Geometry: see drawing. Coordinates: mm, zero at the bounding-box minimum. Give positions to 0.01 mm unless a question says otherwise; leave off trailing zeros. Write each loop counter-clockwise with the first axis right and the second up, starting at its lowest first coordinate (ties: lowest second). Pieces come first, ordered by that corner, then holes. Notation, with made-up numbers: M -24,-38 L -17,-38 A7 ccw -17,-28 Z; hole C 21,67.5 d10. An arc over 180 degrees is marked long. Use a Markdown table: item, result. Add a question column.
1) Section A-A on y = 6. Return the cut outline in (x, z).
2) Section B-B on x = 47. Return the cut outline in (y, z).
3) Pin query (flat end, axial travel): pin 1 (4 mm diameter, centred on y = 4.5, z = 37.5, fed in from -X); pin 2 (2.5 mm diameter, centred on x = 4.5, y = 3.5, fed in from +Z); pin 3 (2.5 mm diameter, centred on x = 97.5, y = 2.5, fed in from -Z). Return the tip coordinate at first contact, or that it passes through.
4) Line query: line 1 (X direction, y = 6.75, z = 55.5); line 2 (Z direction, x = 93, y = 6); line 3 (Z direction, x = 59.5, y = 1.75). Output: solid intervals per line, ascending.
5) Section C-C on z = 156.5. Return the cut outline in (x, y), then the cut area to 3 significant figures.
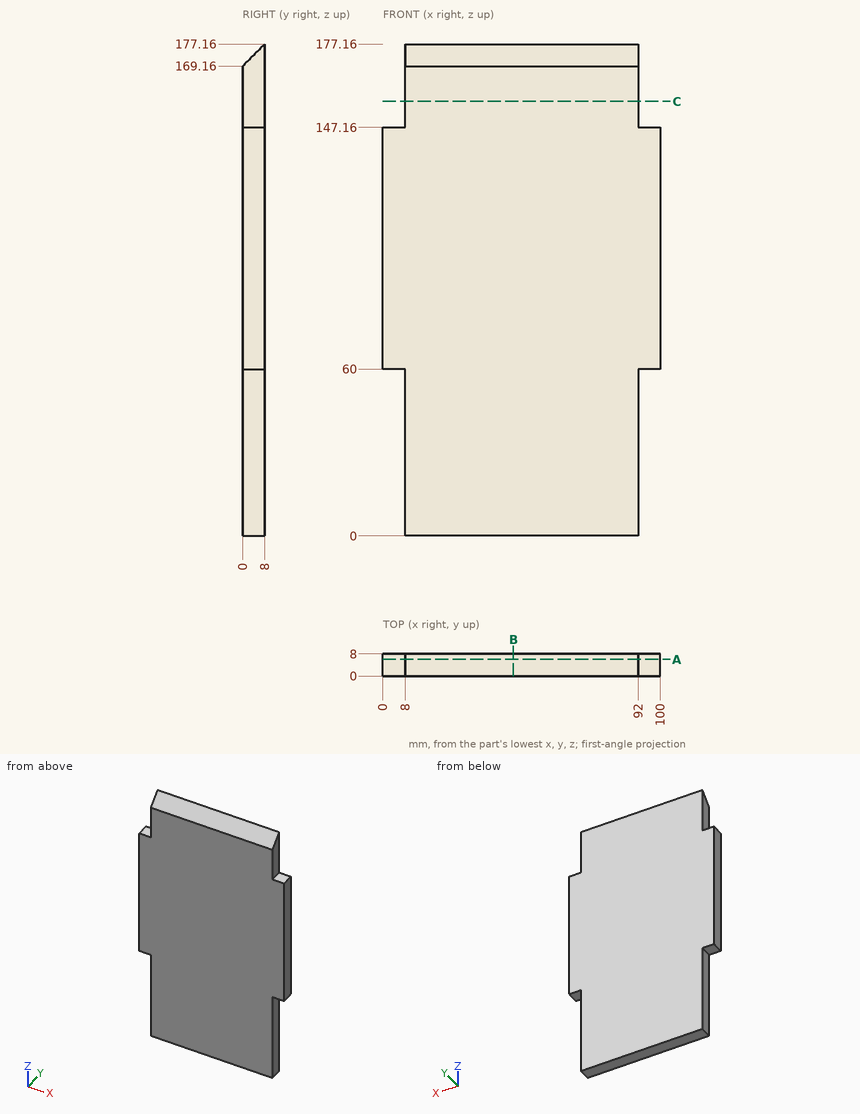
Found:
| question | item | result |
|---|---|---|
| 1 | outline | M 0,60 L 8,60 L 8,0 L 92,0 L 92,60 L 100,60 L 100,147.16 L 92,147.16 L 92,175.16 L 8,175.16 L 8,147.16 L 0,147.16 Z |
| 2 | outline | M 0,0 L 8,0 L 8,177.16 L 0,169.16 Z |
| 3 | pin 1 | x = 8 |
| 3 | pin 2 | z = 147.16 |
| 3 | pin 3 | z = 60 |
| 4 | line 1 | 8 to 92 |
| 4 | line 2 | 60 to 147.16 |
| 4 | line 3 | 0 to 170.91 |
| 5 | outline | M 8,0 L 92,0 L 92,8 L 8,8 Z |
| 5 | area | 672 mm² |
